Input: part model. Units: mm. Frame: model coordinates. Round coordinates to 2 decimals unless told otherwise and drop trailing zeros. Loops run counter-clockwise (first coordinate to the right, second up) from the corner with the lowest first, then second, coordinate; pieces in that order, holes last. Notation, with made-up numbers: (13, -14.5) -> (27, -14.5) arc R27 ccw to (27, 19.5) -> close; hole circle Ø1 at (69.5, -6.5). An arc over 180 degrees is marked (long way). Answer in a Markdown table with one row per item. Add a question column.
Q1. Pin query (flat end, axial travel): pin 1 (5 mm diameter, centred on x = 151, z = 1223.5, fed in from +Y); pin 2 (12 mm diameter, centred on x = -378.5, z = 518.5, fed in from +Y); pin 3 (10 mm diameter, centred on x = -444, z = 423.5, fed in from +Y). Return the tip coordinate at first contact, or that it passes through.
Q2. Ray query, L1, parallel to X at y = 0, z = 301; L2, parallel to X at y = -17.5, z = 263; L3, parallel to Y at x = 409, z = 935. Return the intervals inside material, ascending. Write a range as from..to.
Q3. Section C-C, the plane z = 1050. Output: boundary loops of the cut face in (x, y), and give its area (3 significant figures).
Q4. Section B-B, the plane y = 0. Output: boundary loops of the cut face in (x, z).
Q5. Section A-A, the plane x = 0. Output: boundary loops of the cut face in (y, z), and give its area (3 significant figures).
Q6. Section D-D, the plane x = 444.5. Output: boundary loops of the cut face in (y, z).
Autodesk Inventor part; units mm, degrees
ref_plane "SHELL Plane" through (-428.5067, -428.5067, 0) normal (0.7071, -0.7071, 0) x (0.7071, 0.7071, 0)
ref_plane "ACCESS Plane" through (-213, -1006, 0) normal (0, -1, 0) x (1, 0, 0)
ref_plane "OUTER Plane" through (45, 806, 0) normal (0, 1, 0) x (-1, 0, 0)
sketch "floor angle sketch" plane through (0, 0, 0) normal (0, 0, 1) x (1, 0, 0)
  line L0 (0, 0) -> (0, -240.1382) construction
  line L1 (0, 0) -> (0, -1006)
  line L2 (-428.5067, -428.5067) -> (428.5067, 428.5067) construction
  circle A0 centre (0, 0) radius 606 construction
  line L3 (0, 0) -> (0, 806)
  line L4 (45, 806) -> (-45, 806)
  line L5 (-213, -1006) -> (213, -1006)
  line L6 (0, 0) -> (-309.8702, -851.3615)
  line L7 (0, 0) -> (0, 706)
  line L8 (45, 706) -> (-45, 706)
  line L9 (-370.9503, -829.1302) -> (-248.7902, -873.5928)
  dimension "d51" = 1212
  dimension "d52" = 45
  dimension "d54" = 0
  dimension "d55" = 180
  dimension "d56" = 426
  dimension "d58" = 90
  dimension "d59" = 90
  dimension "d60" = 180
  dimension "d61" = 706
  dimension "d62" = 130
  dimension "d63" = 20
  dimension "d64" = 806
  dimension "d65" = 906
  dimension "d66" = 1006
ref_plane "SHELL Plane" through (-428.5067, -428.5067, 0) normal (0.7071, -0.7071, 0) x (0.7071, 0.7071, 0)
ref_plane "ACCESS Plane" through (-213, -1006, 0) normal (0, -1, 0) x (1, 0, 0)
ref_plane "OUTER Plane" through (45, 806, 0) normal (0, 1, 0) x (-1, 0, 0)
ref_plane "INNER Plane" through (45, 706, 0) normal (0, 1, 0) x (-1, 0, 0)
ref_plane "CHARGE Plane" through (-370.9503, -829.1302, 0) normal (-0.342, -0.9397, 0) x (0.9397, -0.342, 0)
sketch "Sketch13" plane through (-428.5067, -428.5067, 0) normal (0.7071, -0.7071, 0) x (0.7071, 0.7071, 0)
  line L0 (606, 0) -> (606, 892.6829)
  line L1 (0, 0) -> (6, 0)
  line L2 (6, 0) -> (6, 1500)
  line L3 (6, 1500) -> (0, 1500)
  line L4 (0, 1500) -> (0, 0)
  dimension "d75" = 1500
  dimension "d76" = 6
  dimension "d77" = 1212
revolve "Revolution2" add sketch "Sketch13" angle 359.9 about axis through (0, 0, 0) along (0, 0, 1)
sketch "Sketch14" plane through (-213, -1006, 0) normal (0, -1, 0) x (1, 0, 0)
  circle A0 centre (213, 1000) radius 213
  point P0 (213, 0)
  dimension "d79" = 1000
  dimension "d80" = 426
extrude "ACCESS" cut sketch "Sketch14" against normal up to next
sketch "Sketch15" plane through (45, 706, 0) normal (0, 1, 0) x (-1, 0, 0)
  circle A0 centre (45, 270) radius 45
  point P0 (45, 0)
  dimension "d84" = 90
  dimension "d85" = 270
extrude "INNER" cut sketch "Sketch15" against normal up to next
sketch "Sketch16" plane through (45, 806, 0) normal (0, 1, 0) x (-1, 0, 0)
  circle A0 centre (45, 1050) radius 45
  point P0 (45, 0)
  dimension "d88" = 1050
  dimension "d89" = 90
extrude "Extrusion9" cut sketch "Sketch16" against normal up to next
equation "\"BendRadius\" = Thickness"
equation "\"BendReliefWidth\" = Thickness"
equation "\"BendReliefDepth\" = 0.5 * Thickness"
equation "\"CornerReliefSize\" = 4 * Thickness"
equation "\"MinimumRemnant\" = 2 * Thickness"
equation "\"TransitionRadius\" = BendRadius"
equation "\"JacobiRadiusSize\" = BendRadius"
equation "\"GapSize\" = Thickness"
properties part number "TZS 1202 SHELL" material "Steel"
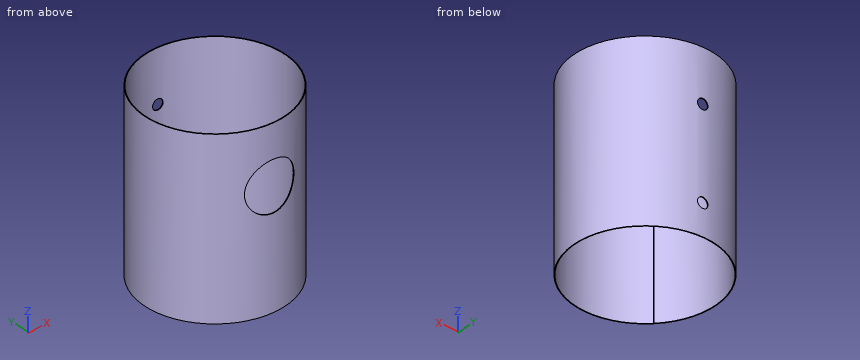
Answer block:
| question | item | result |
|---|---|---|
| 1 | pin 1 | y = 587.52 |
| 1 | pin 2 | y = 478 |
| 1 | pin 3 | y = 417.75 |
| 2 | L1 | -606..-600, 600..606 |
| 2 | L2 | -605.75..-599.74, 599.74..605.75 |
| 2 | L3 | -447.16..-439, 439..447.16 |
| 3 | outline | (-429.25, -427.76) -> (-425, -423.52) arc R600 cw to (-45, 598.31) -> (-45, 604.33) arc R606 ccw to start; (-428.51, -428.51) arc R606 ccw to (-207.05, -569.53) -> (-207.05, -563.14) arc R600 cw to (-424.26, -424.26) -> close; (45, 598.31) arc R600 cw to (207.05, -563.14) -> (207.05, -569.53) arc R606 ccw to (45, 604.33) -> close |
| 3 | area | 19,600 mm^2 |
| 4 | outline | (-606, 0) -> (-600, 0) -> (-600, 1500) -> (-606, 1500) -> close; (600, 0) -> (606, 0) -> (606, 1500) -> (600, 1500) -> close |
| 5 | outline | (-606, 0) -> (-600, 0) -> (-600, 787) -> (-606, 787) -> close; (-606, 1213) -> (-600, 1213) -> (-600, 1500) -> (-606, 1500) -> close; (600, 0) -> (606, 0) -> (606, 225) -> (600, 225) -> close; (600, 315) -> (606, 315) -> (606, 1005) -> (600, 1005) -> close; (600, 1095) -> (606, 1095) -> (606, 1500) -> (600, 1500) -> close |
| 5 | area | 14,400 mm^2 |
| 6 | outline | (-411.89, 0) -> (-403.01, 0) -> (-403.01, 1500) -> (-411.89, 1500) -> close; (403.01, 0) -> (411.89, 0) -> (411.89, 1500) -> (403.01, 1500) -> close |
